from build123d import *

# Parameters (mm, degrees)
PAD_DEPTH = 1.2


with BuildPart() as part:
    # Sketch → Pad (new body)
    with BuildSketch(Plane.XY):
        Polygon((-32.45, -17), (31.15, -17), (31.25, 0), (32.2, 0), (32.45, 17), (-33.75, 17), (-33.5, 0), (-32.55, 0), align=None)
    extrude(amount=PAD_DEPTH)

    # Sketch001 → AdditiveLoft section 0
    with BuildSketch(Plane.XY.offset(1.2)):
        Polygon((32.45, 17), (32.2, 0), (31.25, 0), (31.15, -17), (30.349986, -17), (30.454692, 0.8), (31.411678, 0.8), (31.63815, 16.200086), (-32.93815, 16.200086), (-32.711678, 0.8), (-31.754692, 0.8), (-31.649986, -17), (-32.45, -17), (-32.55, 0), (-33.5, 0), (-33.75, 17), align=None)
    # Sketch002 → AdditiveLoft section 1
    with BuildSketch(Plane.XY.offset(2.4)):
        Polygon((32.45, 17), (32.2, 0), (31.25, 0), (31.15, -17), (30.849995, -17), (30.95176, 0.3), (31.904379, 0.3), (32.145556, 16.700032), (-33.445556, 16.700032), (-33.204379, 0.3), (-32.25176, 0.3), (-32.149995, -17), (-32.45, -17), (-32.55, 0), (-33.5, 0), (-33.75, 17), align=None)
    loft()


solid = part.part
Input: part model. Units: mm. Frame: model coordinates. Give positions to 0.01 mm unless a question says otherwise; leave off trailing zeros. Write each loop counter-clockwise with the first axis right and the second up, starting at its lowest first coordinate (ties: lowest second). Pieces come first, ordered by that corner, then holes. Notation, with made-up numbers: M 1,48.5 L 24,48.5 A26 cw 24,73.5 Z; hole C 78,-22 d4. An arc over 180 degrees is marked long. Use one line per item in the form item = value.
1. Cut plane A-A on z = 0.45. Return loops of the section in (x, y), and give its area (3 significant figures).
Outcome:
outline = M -33.75,17 L -33.5,0 L -32.55,0 L -32.45,-17 L 31.15,-17 L 31.25,0 L 32.2,0 L 32.45,17 Z
area = 2,200 mm²
2. First-contact query: P1, Ø2, axis at x = -17, y = -6.5, coming from the +Z side. Flat tip, straight axial feed; report the tip coordinate or a pass-through.
Outcome:
P1 = 1.2
3. Ray query, L1, parallel to Z at x = -20.5, y = 14; L2, parallel to X at y = 12, z = 2.25; L3, parallel to X at y = -6.5, z = 1.95. Return the intervals inside material, ascending.
Outcome:
L1 = 0 to 1.2
L2 = -33.68 to -33.31, 32.01 to 32.38
L3 = -32.51 to -32.02, 30.72 to 31.21
